Can you work these out from the model? Positions are in its coordinate system, mm. A direction names the side the tool comes from. Coordinates: 2 decimals unless noted, no trailing zeros. Order: outer loops, then holes, each group sorted by start corner. A loop starts at its lowest first (then second) coordinate and runs counter-clockwise, first axis right, second up. Notation, with made-up numbers: (76.5, -25.5) -> (122.5, -25.5) arc R12 ccw to (122.5, -16.5) -> close; hole circle Ø5 at (31.25, 39.5). An arc over 180 degrees is marked (long way). Answer in a Markdown table with one row per item.
Autodesk Inventor part; units mm, degrees
ref_plane "Work Plane1" through (15, 0, 0) normal (1, 0, 0) x (0, 0, -1)
ref_plane "YZ Plane" through (0, 0, 0) normal (1, 0, 0) x (0, 1, 0)
ref_plane "XZ Plane" through (0, 0, 0) normal (0, 1, 0) x (-1, 0, 0)
sketch "Sketch1" plane through (0, 0, 0) normal (1, 0, 0) x (0, 1, 0)
  circle A0 centre (0, 0) radius 4
  circle A1 centre (0, 0) radius 5
  dimension "d0" = 8
  dimension "d1" = 10
extrude "Extrusion1" add sketch "Sketch1" along normal blind 20
ref_plane "Work Plane1" through (15, 0, 0) normal (1, 0, 0) x (0, 0, -1)
sketch "Sketch2" plane through (15, 0, 0) normal (1, 0, 0) x (0, 0, -1)
  circle A0 centre (0, 0) radius 4
extrude "Extrusion2" add sketch "Sketch2" along normal blind 85
sketch "Sketch3" plane through (0, 0, 0) normal (0, 1, 0) x (-1, 0, 0)
  line L0 (0, 0) -> (-7.5, 0)
  circle A0 centre (-7.5, 0) radius 1.5
  dimension "d7" = 7.5
  dimension "d8" = 3
extrude "Extrusion3" cut sketch "Sketch3" against normal blind 60
thread "Thread1"
sketch "Sketch4" plane through (0, 0, 0) normal (0, 0, 1) x (1, 0, 0)
  line L0 (100, -4) -> (100, 4)
  line L1 (100, 0) -> (90, 0)
  circle A0 centre (90, 0) radius 2
  point P0 (0, 0)
  dimension "d13" = 10
  dimension "d14" = 4
extrude "Extrusion4" cut sketch "Sketch4" along normal blind 10
sketch "Sketch5" plane through (90, 0, 0) normal (0, 0, 1) x (1, 0, 0)
  circle A0 centre (0, 0) radius 2
  point P0 (-90, 0)
extrude "Extrusion5" add sketch "Sketch5" along normal blind 2
chamfer "Chamfer1" distance 0.5 angle 45 1 edges at (88.0001, -0.0148, 4)
sketch "Sketch6" plane through (100, 0, 0) normal (1, 0, 0) x (0, 0, -1)
  circle A0 centre (0, 0) radius 4
extrude "Extrusion6" add sketch "Sketch6" along normal blind 2
properties part number "4x2020_axis" material "Stainless Steel"
(1) Suppose I cut it at B-B (x = 28). Please give me the cut outline in (y, z).
Response values:
| item | result |
|---|---|
| outline | circle Ø8 at (0, 0) |
(2) Suppose I cut it at A-A (z = 0). Please give me the cut outline in (x, y), and give its area (3 significant figures).
Response values:
| item | result |
|---|---|
| outline | (0, -5) -> (6, -5) -> (6, -4) -> (0, -4) -> close; (0, 4) -> (15, 4) -> (15, -4) -> (9, -4) -> (9, -5) -> (20, -5) -> (20, -4) -> (102, -4) -> (102, 4) -> (20, 4) -> (20, 5) -> (0, 5) -> close |
| area | 733 mm2 |
(3) I need wall thicknesses on line 1 (Z direction, x = 9.25, y = 0); line 2 (X direction, y = 0, z = 2.75); line 3 (X direction, y = -3.5, z = -2.5). Which ranges of each line are inside material? Lowest first, please. Write a range as [from, to].
Response values:
| item | result |
|---|---|
| line 1 | [-5, -4], [4, 5] |
| line 2 | [15, 88], [92, 102] |
| line 3 | [0, 20] |
(4) On a 3-axis mill with a long thin cutter (end or side, diameter ignored), from which of +Z, -Z, +X, -X, +Y, -Y can I reach the whole of each face in a straight line? I mean faces 1 (the cylindrical face through (60.426, 1.532, -3.695)), 2 (the flat face through (15, 0, 0)), 3 (the cylindrical face through (89.74, -1.983, 2.573)), 4 (the flat face through (102, 0, 0)). Say none if no direction works.
Response values:
| item | result |
|---|---|
| face 1 | +X |
| face 2 | -X |
| face 3 | +Z |
| face 4 | +Z, -Z, +X, +Y, -Y |
(5) Suppose I cut it at C-C (x = 7.5). Please give me the cut outline in (y, z).
Response values:
| item | result |
|---|---|
| outline | (-4.77, -1.5) arc R5 ccw (long way) to (-4.77, 1.5) -> (-3.71, 1.5) arc R4 cw (long way) to (-3.71, -1.5) -> close |
(6) Will these pins go through, and if not, where does the flat tip stop? pin 1 Ø3 at (x, y) = (90, 0) entering from +Z; pin 2 Ø1 at (y, z) = (-0.5, -3) entering from -X; pin 3 Ø4 at (x, y) = (82.5, -2) entering from +Z.
Response values:
| item | result |
|---|---|
| pin 1 | z = 2 |
| pin 2 | x = 15 |
| pin 3 | z = 4 |
(7) We'd pull the mould along Z, two halves only. Please class faces 5 (the cylindrical face through (9.86, 4.619, 1.915)), 6 (the cylindrical face through (7.395, 3.695, 1.532)), 7 (the flat face through (90, 0, 2)), 8 (the cylindrical face through (7.825, -4.345, -1.464)): +Z half, -Z half, draft (parallel to the pull), parting line (faces both ways), or undercut.
Response values:
| item | result |
|---|---|
| face 5 | parting line |
| face 6 | undercut |
| face 7 | +Z half |
| face 8 | undercut |
